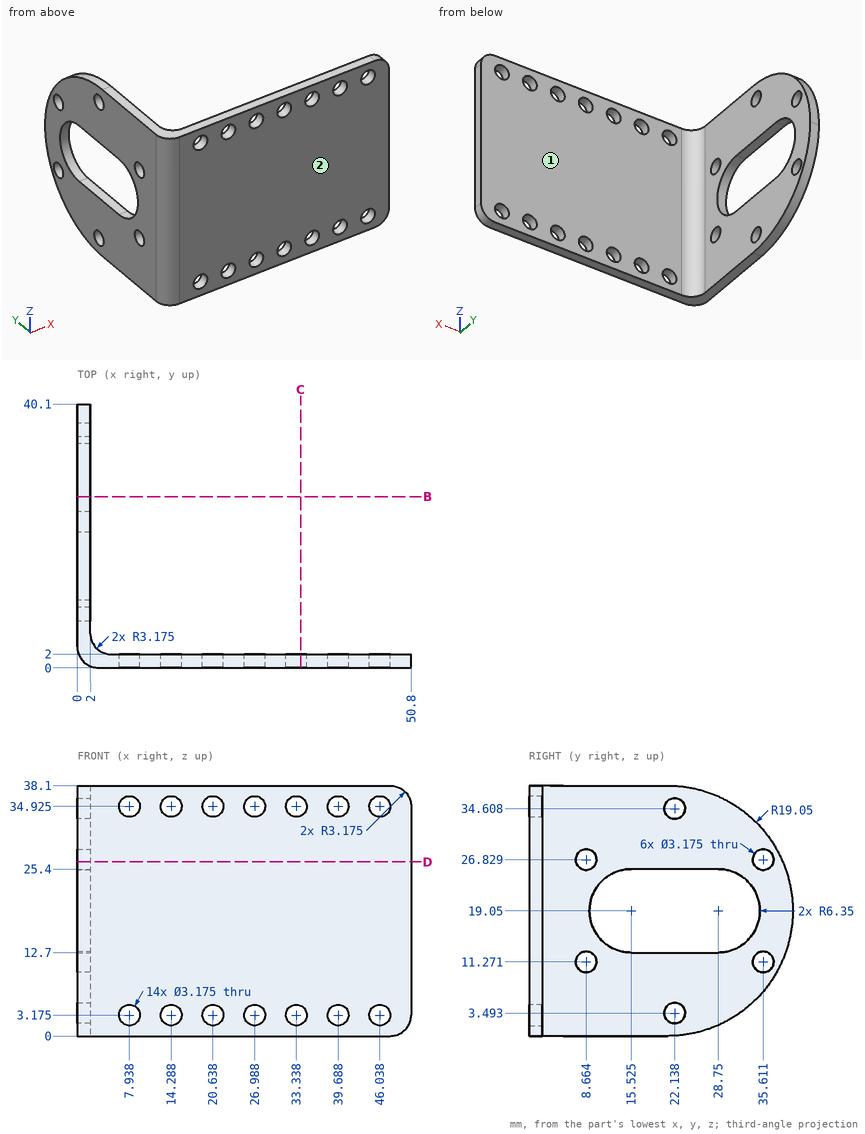
Input: dimensioned drawing with shaded views. Units: mm. Origin: part minimum x, y, z. A direction names the side the tool comes from. Round coordinates to 2 decimals unless told otherwise and drop trailing zeros. Order: outer loops, then holes, each group sorted by start corner. A loop starts at its lowest first (then second) coordinate and runs counter-clockwise, first axis right, second up. Notation, with made-up numbers: (-18.5, 81.25) -> (29.5, 81.25) arc R9 cw to (29.5, 86.25) -> close; hole circle Ø10 at (-11, 20.5). An arc over 180 degrees is marked (long way). Put each result on its own line as item: value. Start each with the question number.
Q1. Reachability of the marked faces 1 and 2 from +Z, -Z, +X, -X, +Y, -Y: full face, straight path, thin tool, end or side. Return the list, or none.
Q2. Section B-B on y = 26. Return the cut outline in (x, z) (1 decimal).
Q3. Section D-D on z = 26.5. Give the number of separate pieces and of enclosed holes in the cut face.
Q4. Line query: probe 1 along X at (y, z) = (38, 23); probe 2 along Y at (x, z) = (4, 27) (1 decimal). Output: solid intervals per line, ascending.
Q5. First-contact query: pin 1 (4 mm diameter, centred on y = 35.61, z = 11.27, fed in from +X); pin 2 (3.5 mm diameter, centred on x = 26.99, z = 34.93, fed in from +Y). Flat tips, straight axial feed; report the tip coordinate or a pass-through.
Q6. Section C-C on x = 34. Return the cut outline in (y, z).
Ans:
1. face 1: +Z, -Z, +X, +Y
1. face 2: +Z, -Z, +X, -X, -Y
2. outline: (0, 0.7) -> (2, 0.7) -> (2, 12.7) -> (0, 12.7) -> close; (0, 25.4) -> (2, 25.4) -> (2, 37.4) -> (0, 37.4) -> close
3. separate pieces: 3
3. enclosed holes: 0
4. probe 1: x = 0 to 2
4. probe 2: y = 0 to 2.2
5. pin 1: stops at x = 2
5. pin 2: stops at y = 2
6. outline: (0, 0) -> (2, 0) -> (2, 1.73) -> (0, 1.73) -> close; (0, 4.62) -> (2, 4.62) -> (2, 33.48) -> (0, 33.48) -> close; (0, 36.37) -> (2, 36.37) -> (2, 38.1) -> (0, 38.1) -> close
